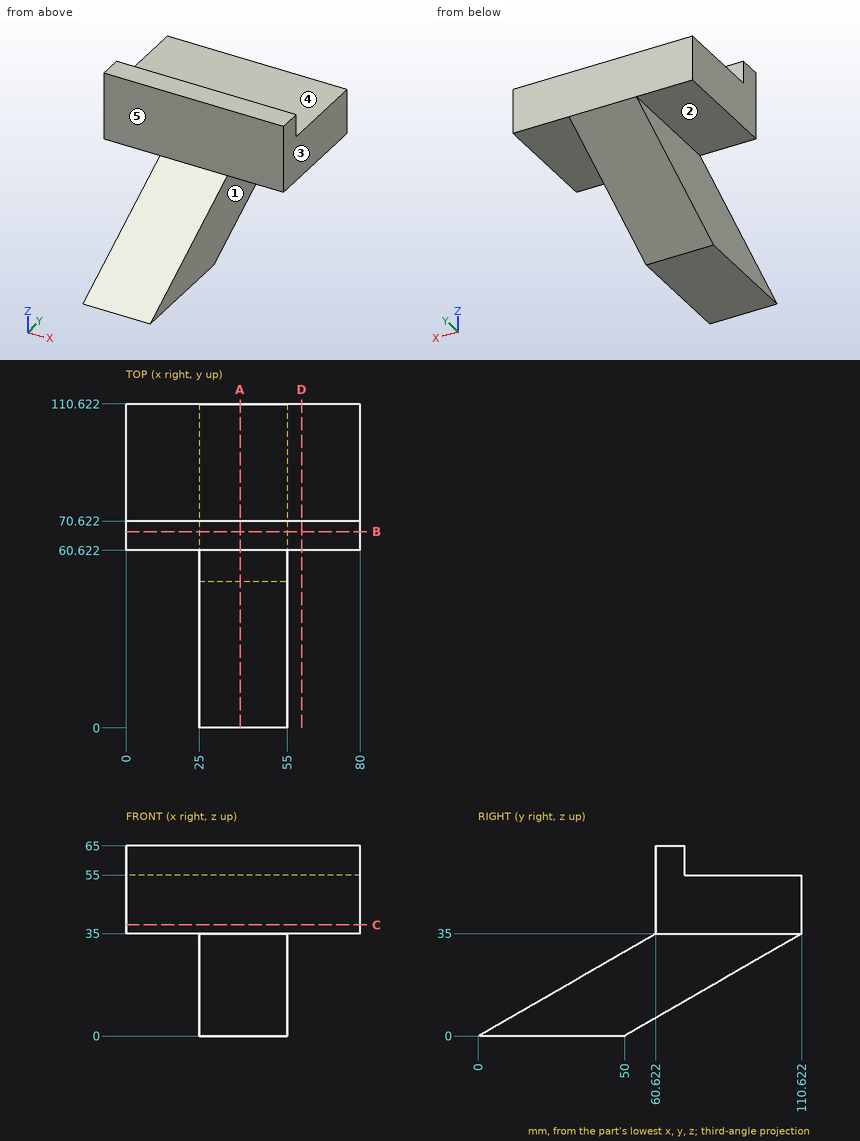
Source: three-view drawing plus pictorial views. Frame: mm from the lowest corner of the part. A direction names the side the tool comes from. Round coordinates to 2 decimals unless told otherwise and drop trailing zeros. Write each loop counter-clockwise with the first axis right and the second up, starting at its lowest first coordinate (ties: lowest second). Pieces come first, ordered by that corner, then holes. Notation, with made-up numbers: M 48.25,47 L 100.25,47 A19 cw 100.25,52 Z; hole C 33,-25 d2. An arc over 180 degrees is marked long. Use CSV: the item, a comma, the result in double quotes. Start each with the question number.
Q1. Cut plane A-A on x = 39. Output: boundary loops of the cut face in (y, z).
Q2. Cut plane C-C on z = 38. Output: boundary loops of the cut face in (x, y).
Q3. Access query for the marked faces 1, 2, 3, 4 and 5. Directions: +Z, -Z, +X, -X, +Y, -Y. A direction counts if a zero-diameter tool reaches every point of the face in a straight line with its end or side. Return the directions, or none.
Q4. Cut plane D-D on x = 60. Output: boundary loops of the cut face in (y, z), plus the area to 3 significant figures.
Q5. First-contact query: P1, Ø8, axis at x = 50.5, z = 61, coming from the +Y side; P2, Ø9, axis at x = 57, z = 50, coming from the -Y side; P3, Ø7.5, axis at x = 68.5, y = 86.5, coming from the -Z side. Flat tips, straight axial feed; report the tip coordinate or a pass-through.
Q6. Cut plane B-B on y = 67. Output: boundary loops of the cut face in (x, z) (3 decimals), plus the area to 3 significant figures.
Q7. Line query: line 1 (Y direction, x = 16, z = 39); line 2 (Y direction, x = 45.5, z = 61); line 3 (X direction, y = 42.5, z = 19.5). Output: solid intervals per line, ascending. Write a range as from..to.
Results found:
1,outline,"M 0,0 L 50,0 L 110.62,35 L 110.62,55 L 70.62,55 L 70.62,65 L 60.62,65 L 60.62,35 Z"
2,outline,"M 0,60.62 L 80,60.62 L 80,110.62 L 0,110.62 Z"
3,face 1,"-Z, +X, +Y, -Y"
3,face 2,"-Z, -X, +Y, -Y"
3,face 3,"+Z, -Z, +X, +Y, -Y"
3,face 4,"+Z, +X, -X, +Y"
3,face 5,"+Z, +X, -X, -Y"
4,outline,"M 60.62,35 L 110.62,35 L 110.62,55 L 70.62,55 L 70.62,65 L 60.62,65 Z"
4,area,"1,100 mm^2"
5,P1,"y = 70.62"
5,P2,"y = 60.62"
5,P3,"z = 35"
6,outline,"M 0,35 L 25,35 L 25,9.815 L 55,9.815 L 55,35 L 80,35 L 80,65 L 0,65 Z"
6,area,"3,160 mm^2"
7,line 1,"60.62..110.62"
7,line 2,"60.62..70.62"
7,line 3,"25..55"
